Model file for the job. Use its own axes, mm. Face numbers are marked on the shaded views. A direction names the side the tool comes from. Coordinates: 2 decimals unless noted, no trailing zeros. Order: outer loops, then holes, each group sorted by start corner. A loop starts at its lowest first (then second) coordinate and runs counter-clockwise, first axis right, second up. Notation, with made-up numbers: M -39.75,0.25 L -1.75,0.25 A31 cw -1.75,34.25 Z; hole C -34.5,-2 d5. An arc over 180 degrees is marked long. Return JSON: item names as keys, results as strings.
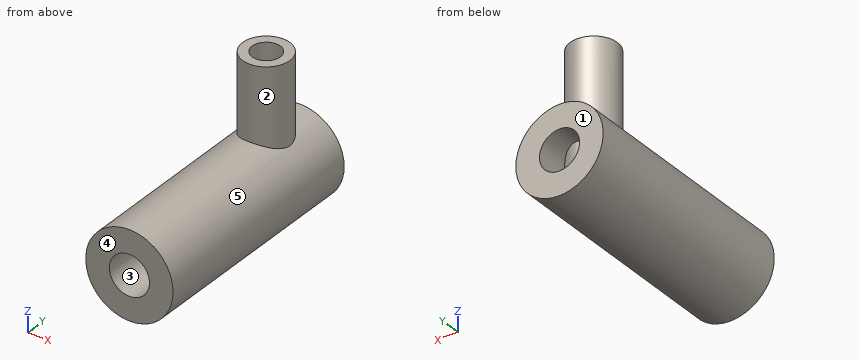
```python
from build123d import *

# Parameters (mm, degrees)
F0_R     = 9.25
F0_R_2   = 4.25
F1_DEPTH = 25
F2_R     = 5
F2_R_2   = 3
F3_DEPTH = 25


with BuildPart() as f1:
    # F0 (on Front) → F1 (new body, symmetric)
    with BuildSketch(Plane.XZ):
        Circle(F0_R)
        Circle(F0_R_2, mode=Mode.SUBTRACT)
    extrude(amount=F1_DEPTH, both=True)

    # F2 (on Top) → F3 (join)
    with BuildSketch(Plane.XY):
        with Locations((0, 15)):
            Circle(F2_R)
        with Locations((0, 15)):
            Circle(F2_R_2, mode=Mode.SUBTRACT)
    extrude(amount=F3_DEPTH)


solid = f1.part
```
Item 1: 3-axis set-ups, long thin cutter, end or side, ignore diameter. For the marked faces 1 and 2: which of +Z, -Z, +X, -X, +Y, -Y reach the whole face in a straight line?
Check result:
{"face 1": "+Z, -Z, +X, -X, +Y", "face 2": "+Z"}
Item 2: Saw through at B-B (y = 19). Write the cut outline in (x, z), and give its area (3 significant figures).
Check result:
{"outline": "M -3,8.75 A9.25 ccw long 3,8.75 L 3,25 L -3,25 Z; hole M -3,0 L -3,3.01 A4.25 ccw long 3,3.01 L 3,0 Z", "area": "331 mm2"}
Item 3: Pull direction Z, two halves, no side cores. Call the marked faces 3, 4 and 5: +Z half, -Z half, draft (parallel to the pull), parting line (faces both ways), or undercut.
Check result:
{"face 3": "undercut", "face 4": "draft", "face 5": "parting line"}
Item 4: Wall check: line 1 (Y direction, x = 0, z = 14); line 2 (X direction, y = 15, z = 14); line 3 (Z direction, x = 0, y = -13.5). Give the ranges that are in metal, low to high.
Check result:
{"line 1": "y = 10 to 12, 18 to 20", "line 2": "x = -5 to -3, 3 to 5", "line 3": "z = -9.25 to -4.25, 4.25 to 9.25"}
Item 5: Saw through at C-C (z = -1.5). Write the cut outline in (x, y).
Check result:
{"outline": "M -9.13,-25 L -3.98,-25 L -3.98,25 L -9.13,25 Z; M 3.98,-25 L 9.13,-25 L 9.13,25 L 3.98,25 Z"}
Item 6: Saw through at A-A (x = 0). Write the cut outline in (y, z), and give its area (3 significant figures).
Check result:
{"outline": "M -25,-9.25 L 25,-9.25 L 25,-4.25 L -25,-4.25 Z; M -25,4.25 L 10,4.25 L 10,0 L 12,0 L 12,4.25 L 18,4.25 L 18,0 L 20,0 L 20,4.25 L 25,4.25 L 25,9.25 L 20,9.25 L 20,25 L 18,25 L 18,9.25 L 12,9.25 L 12,25 L 10,25 L 10,9.25 L -25,9.25 Z", "area": "580 mm2"}
Item 7: Saw through at D-D (z = 15.5). Write the cut outline in (x, y), and give its area (3 significant figures).
Check result:
{"outline": "C 0,15 d10; hole C 0,15 d6", "area": "50.3 mm2"}
Item 8: Drop flat-ended pins along their axis: pin 1 Ø5 at (x, z) = (-4, 21.5) entering from -Y; pin 2 Ø5 at (x, y) = (4.5, -11) entering from -Z; pin 3 Ø1.5 at (y, z) = (-11.5, 5.5) entering from +X. Give the stop position or say it passes through.
Check result:
{"pin 1": "stops at y = 10.23", "pin 2": "stops at z = -9.03", "pin 3": "stops at x = 7.94"}
